Input: dimensioned drawing with shaded views. Units: mm. Origin: part minimum x, y, z. Give positions to 0.01 mm unless a question says otherwise; leave off trailing zeros. Write each loop counter-clockwise with the first axis right and the second up, starting at its lowest first coordinate (ties: lowest second). Pieces come first, ordered by that corner, then holes. Notation, with made-up numbers: (-5.5, 32.25) -> (24.5, 32.25) arc R30 ccw to (24.5, 61.25) -> close; hole circle Ø9 at (3.5, 38.5). An arc over 180 degrees is marked (long way). Answer in a Markdown table with one row per item. Add a question column.
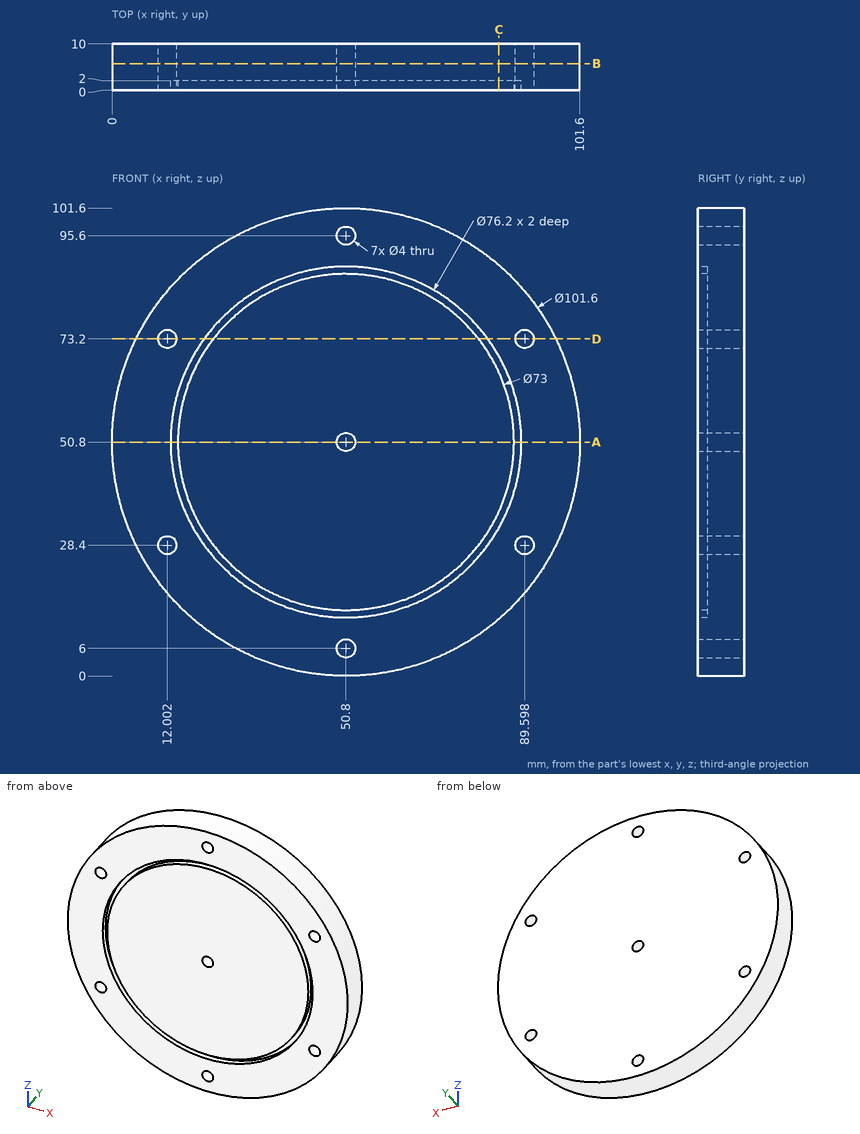
Q1. Section B-B on y = 5.75. Return loops of the section in (x, z).
Q2. Section A-A on z = 50.8. Return loops of the section in (x, y).
Q3. Section D-D on z = 73.2. Return loops of the section in (x, y), and give its area (3 significant figures).
Q4. Section C-C on x = 84. Return loops of the section in (y, z).
Q5. Line query: probe 1 along Z at (x, y) = (50.8, 7.75); probe 2 along X at (y, z) = (5, 50.8); probe 3 along X at (y, z) = (5.75, 73.2). Output: solid intervals per line, ascending. Write a range as from..to.
Q6. Contact query for flat-ended pins moving along their axis: pin 1 Ø6.5 at (x, z) = (50.8, 95.6) entering from +Y; pin 2 Ø6 at (y, z) = (5.5, 70.5) entering from +X; pin 3 Ø2.5 at (x, z) = (50.8, 50.8) entering from +Y; pin 4 Ø1.5 at (y, z) = (4, 48.5) entering from +X. Output: stop coordinate, or through.
Checks:
| question | item | result |
|---|---|---|
| 1 | outline | circle Ø101.6 at (50.8, 50.8); hole circle Ø4 at (12, 28.4); hole circle Ø4 at (12, 73.2); hole circle Ø4 at (50.8, 6); hole circle Ø4 at (50.8, 50.8); hole circle Ø4 at (50.8, 95.6); hole circle Ø4 at (89.6, 28.4); hole circle Ø4 at (89.6, 73.2) |
| 2 | outline | (0, 0) -> (12.7, 0) -> (12.7, 2) -> (14.3, 2) -> (14.3, 0) -> (48.8, 0) -> (48.8, 10) -> (0, 10) -> close; (52.8, 0) -> (87.3, 0) -> (87.3, 2) -> (88.9, 2) -> (88.9, 0) -> (101.6, 0) -> (101.6, 10) -> (52.8, 10) -> close |
| 3 | outline | (5.21, 0) -> (10, 0) -> (10, 10) -> (5.21, 10) -> close; (14, 0) -> (19.98, 0) -> (19.98, 2) -> (21.98, 2) -> (21.98, 0) -> (79.62, 0) -> (79.62, 2) -> (81.62, 2) -> (81.62, 0) -> (87.6, 0) -> (87.6, 10) -> (14, 10) -> close; (91.6, 0) -> (96.39, 0) -> (96.39, 10) -> (91.6, 10) -> close |
| 3 | area | 824 mm^2 |
| 4 | outline | (0, 12.35) -> (10, 12.35) -> (10, 89.25) -> (0, 89.25) -> (0, 69.49) -> (2, 69.49) -> (2, 65.97) -> (0, 65.97) -> (0, 35.63) -> (2, 35.63) -> (2, 32.11) -> (0, 32.11) -> close |
| 5 | probe 1 | 0..4, 8..48.8, 52.8..93.6, 97.6..101.6 |
| 5 | probe 2 | 0..48.8, 52.8..101.6 |
| 5 | probe 3 | 5.21..10, 14..87.6, 91.6..96.39 |
| 6 | pin 1 | y = 10 |
| 6 | pin 2 | x = 98.78 |
| 6 | pin 3 | through |
| 6 | pin 4 | x = 101.58 |
